Autodesk Fusion 360 part; units mm, degrees
sketch "Sketch1" plane through (0, 0, 0) normal (0, 1, 0) x (1, 0, 0)
  line L0 (0, 0) -> (-735.0705, 0) construction
  line L1 (0, 0) -> (-636.5897, -367.5353) construction
  line L2 (0, 0) -> (-735.0705, -196.9616) construction
  circle A0 centre (-735.0705, -196.9616) radius 25
  circle A1 centre (-735.0705, -196.9616) radius 12.5
  circle A2 centre (-700.3409, 0) radius 25
  circle A3 centre (-700.3409, 0) radius 12.5
  circle A4 centre (-666.6665, -384.9001) radius 25
  circle A5 centre (-666.6665, -384.9001) radius 12.5
  line L3 (-675.7207, -4.3412) -> (-710.4503, -201.3028)
  line L4 (-759.6907, -192.6203) -> (-724.9611, 4.3412)
  line L5 (-643.1742, -376.3496) -> (-711.5782, -188.411)
  line L6 (-690.1588, -393.4506) -> (-758.5628, -205.5121)
  line L7 (-666.6665, -384.9001) -> (-735.0705, -196.9616) construction
  line L8 (-735.0705, -196.9616) -> (-700.3409, 0) construction
  line L9 (-735.0705, -196.9616) -> (-735.0705, 0) construction
  line L10 (-735.0705, -196.9616) -> (-636.5897, -367.5353) construction
  dimension "d2" = 30
  dimension "d3" = 15
  dimension "d6" = 50
  dimension "d7" = 25
  dimension "d8" = 50
  dimension "d9" = 25
  dimension "d10" = 50
  dimension "d11" = 25
  dimension "d15" = 10
  dimension "d16" = 10
  dimension "d17" = 200
extrude "Extrude1" add sketch "Sketch1" along normal mid plane 20
equation "d3 = d2 / 2"
equation "d7 = d6 / 2"
equation "d8 = d6"
equation "d9 = d7"
equation "d10 = d6"
equation "d11 = d7"
equation "d16 = d15"

Autodesk Fusion 360 part; units mm, degrees
sketch "Sketch1" plane through (0, 0, 0) normal (0, 1, 0) x (1, 0, 0)
  line L0 (0, 0) -> (-735.0705, 0) construction
  line L1 (0, 0) -> (-636.5897, -367.5353) construction
  line L2 (0, 0) -> (-735.0705, -196.9616) construction
  circle A0 centre (-769.8001, 0) radius 25
  circle A1 centre (-606.513, -350.1704) radius 25
  circle A2 centre (-735.0705, -196.9616) radius 12.5
  circle A3 centre (-735.0705, -196.9616) radius 25
  line L3 (-759.6907, -201.3028) -> (-794.4203, -4.3412)
  line L4 (-710.4503, -192.6203) -> (-745.18, 4.3412)
  line L5 (-587.3619, -334.1007) -> (-715.9194, -180.8919)
  line L6 (-625.6641, -366.2401) -> (-754.2216, -213.0312)
  circle A4 centre (-769.8001, 0) radius 12.5
  circle A5 centre (-606.513, -350.1704) radius 12.5
  line L7 (-735.0705, 0) -> (-735.0705, -196.9616) construction
  line L8 (-636.5897, -367.5353) -> (-735.0705, -196.9616) construction
  line L9 (-735.0705, -196.9616) -> (-769.8001, 0) construction
  line L10 (-735.0705, -196.9616) -> (-606.513, -350.1704) construction
  dimension "d2" = 30
  dimension "d3" = 15
  dimension "d7" = 50
  dimension "d8" = 50
  dimension "d9" = 25
  dimension "d10" = 50
  dimension "d11" = 25
  dimension "d12" = 25
  dimension "d18" = 10
  dimension "d19" = 10
  dimension "d20" = 200
extrude "Extrude1" add sketch "Sketch1" along normal mid plane 20
equation "d2 = ( 90 / 3 ) * 1 deg"
equation "d3 = d2 / 2"
equation "d8 = d7"
equation "d9 = d7 / 2"
equation "d10 = d7"
equation "d11 = d9"
equation "d12 = d9"
equation "d19 = d18"
Verification items for the finished model (mm, model axes). Round coordinates to 2 decimals unless told otherwise and drop trailing zeros. Write each loop counter-clockwise with the first axis right and the second up, starting at its lowest first coordinate (ties: lowest second). Pieces come first, ordered by that corner, then holes. Notation, with made-up numbers: (48, 21.5) -> (91, 21.5) arc R26 ccw to (91, 50.5) -> close; hole circle Ø1 at (-20.75, 87). An arc over 180 degrees is marked (long way). Write each question's results on one line, items separated by ' | '. Start each with the question number.
1. Draft check along Z on faces 1 (the cylindrical face through (-590.026, -0.14, 368.964)), 2 (the cylindrical face through (-737.78, -0.14, 184.76)), 3 (the cylindrical face through (-757.69, -0.14, 207.61)), 4 (the flat face through (-728.162, -0.14, 92.174)). Enter one of: +Z half, -Z half, draft (parallel to the pull), parting line (faces both ways), or undercut.
2. Material ranges on probe 1 along X at (y, z) = (-3.5, 359.5); probe 2 along X at (y, z) = (-3, 0); probe 3 along Z at (x, y) = (-624, -2), recorded low to high. Write a range as from..to.
3. Cross-section at A-A (y = -1). Enter the section's corners in (x, z), then the cut area to 3 significant figures.
4. Cross-section at D-D (z = 148). Enter the section's corners in (x, y), then the cut area to 3 significant figures.
5. Cross-section at B-B (z = 0). Enter the section's corners in (x, y).
6. Cross-section at C-C (x = -657). Enter the section's corners in (y, z).
7. Depth check by flat-ended pin: P1, Ø6, axis at y = 1, z = 197.5, coming from the -X side; P2, Ø4, axis at y = 8, z = 233, coming from the -X side; P3, Ø10, axis at x = -747, y = -7.5, coming from the -Z side; P4, Ø20, axis at x = -769.8, z = 0, coming from the -Y side. Enter the tip coordinate at first touch or a pass-through.
Solutions:
1) face 1: parting line | face 2: undercut | face 3: +Z half | face 4: -Z half
2) probe 1: x = -631.32..-614.83, -598.19..-583.32 | probe 2: x = -794.8..-782.3, -757.3..-744.41 | probe 3: z = 290.44..368.04
3) outline: (-794.42, 4.34) arc R25 ccw to (-745.18, -4.34) -> (-711.61, 186.02) -> (-587.36, 334.1) arc R25 ccw to (-625.66, 366.24) -> (-754.22, 213.03) arc R25 ccw to (-759.69, 201.3) -> close; hole circle Ø25 at (-769.8, 0); hole circle Ø25 at (-735.07, 196.96); hole circle Ø25 at (-606.51, 350.17) | area: 20,500 mm2
4) outline: (-769.09, -10) -> (-718.32, -10) -> (-718.32, 10) -> (-769.09, 10) -> close | area: 1,020 mm2
5) outline: (-794.8, -10) -> (-782.3, -10) -> (-782.3, 10) -> (-794.8, 10) -> close; (-757.3, -10) -> (-744.41, -10) -> (-744.41, 10) -> (-757.3, 10) -> close
6) outline: (-10, 251.11) -> (10, 251.11) -> (10, 328.9) -> (-10, 328.9) -> close
7) P1: stops at x = -760.89 | P2: stops at x = -739.14 | P3: stops at z = -17.55 | P4: passes through
